```python
from build123d import *

# Parameters (mm, degrees)
SKETCH_1_R          = 12
EXTRUDE_1_DEPTH     = 19
EXTRUDE_START       = -1
SKETCH_2_R          = 2
EXTRUDE_2_DEPTH     = 1
SKETCH_3_R          = 3.5
EXTRUDE_3_DEPTH     = 1.5
SKETCH_4_R          = 2.5
EXTRUDE_4_DEPTH     = 6
CUT_EXTRUDE_START   = -5.7
CUT_EXTRUDE_1_DEPTH = 5.7
EXTRUDE_START_2     = -16.3
EXTRUDE_5_DEPTH     = 16.3
CHAMFER_1_SIZE      = 1
FILLET_1_R          = 1
CUT_EXTRUDE_2_DEPTH = 2
SKETCH_8_R          = 0.5
EXTRUDE_6_DEPTH     = 13


with BuildPart() as part:
    # Эскиз1 → Бобышка-Вытянуть1 (new body)
    with BuildSketch(Plane.XY):
        Circle(SKETCH_1_R)
    extrude(amount=EXTRUDE_1_DEPTH)

    # Эскиз2 → Бобышка-Вытянуть2 (add)
    # profile 1 of 2: a face of its own
    with BuildSketch(Plane.XY.offset(19).offset(EXTRUDE_START)):
        with BuildLine():
            Line((-15.5, 3.5), (-11.478240283, 3.5))
            ThreePointArc((-11.478240283, 3.5), (-12, 0), (-11.478240283, -3.5))
            Line((-11.478240283, -3.5), (-15.5, -3.5))
            ThreePointArc((-15.5, -3.5), (-19, 0), (-15.5, 3.5))
        make_face()
        with Locations((-15.5, 0)):
            Circle(SKETCH_2_R, mode=Mode.SUBTRACT)
    # profile 2 of 2: a face of its own
    with BuildSketch(Plane.XY.offset(19).offset(EXTRUDE_START)):
        with BuildLine():
            Line((15.5, -3.5), (11.478240283, -3.5))
            ThreePointArc((11.478240283, -3.5), (12, 0), (11.478240283, 3.5))
            Line((11.478240283, 3.5), (15.5, 3.5))
            ThreePointArc((15.5, 3.5), (19, 0), (15.5, -3.5))
        make_face()
        with Locations(Location((15.5, 0, 0), (0, 0, 180))):
            Circle(SKETCH_2_R, mode=Mode.SUBTRACT)
    extrude(amount=EXTRUDE_2_DEPTH)

    # Эскиз3 → Бобышка-Вытянуть3 (add)
    with BuildSketch(Plane.XY.offset(19)):
        with Locations((0, 6.5)):
            Circle(SKETCH_3_R)
    extrude(amount=EXTRUDE_3_DEPTH)

    # Эскиз4 → Бобышка-Вытянуть4 (add)
    with BuildSketch(Plane.XY.offset(20.5)):
        with Locations((0, 6.5)):
            Circle(SKETCH_4_R)
    extrude(amount=EXTRUDE_4_DEPTH)

    # Эскиз5 → Вырез-Вытянуть1 (cut)
    with BuildSketch(Plane.XY.offset(26.5).offset(CUT_EXTRUDE_START)):
        with BuildLine():
            Line((-1.5, 8.5), (-1.5, 4.5))
            ThreePointArc((-1.5, 4.5), (-2.5, 6.5), (-1.5, 8.5))
        make_face()
        with BuildLine():
            Line((1.5, 8.5), (1.5, 4.5))
            ThreePointArc((1.5, 4.5), (2.5, 6.5), (1.5, 8.5))
        make_face()
    extrude(amount=CUT_EXTRUDE_1_DEPTH, mode=Mode.SUBTRACT)

    # Эскиз6 → Бобышка-Вытянуть5 (add)
    with BuildSketch(Plane.XY.offset(19).offset(EXTRUDE_START_2)):
        with BuildLine():
            Line((-7.5, -16.5), (7.5, -16.5))
            Line((7.5, -16.5), (7.5, -9.367496998))
            ThreePointArc((7.5, -9.367496998), (0, -12), (-7.5, -9.367496998))
            Line((-7.5, -9.367496998), (-7.5, -16.5))
        make_face()
    extrude(amount=EXTRUDE_5_DEPTH)

    # Фаска1
    chamfer_1_edges = [part.edges().sort_by_distance(p)[0] for p in [
        (-7.5, -16.5, 10.85),
        (7.5, -16.5, 10.85),
    ]]
    chamfer(chamfer_1_edges, length=CHAMFER_1_SIZE)

    # Скругление1
    fillet_1_edges = [part.edges().sort_by_distance(p)[0] for p in [
        (-12, 0, 0),
    ]]
    fillet(fillet_1_edges, radius=FILLET_1_R)

    # Эскиз7 → Вырез-Вытянуть2 (cut)
    with BuildSketch(Plane.XZ.offset(16.5)):
        with BuildLine():
            Line((-3.5, 15.6), (3.5, 15.6))
            ThreePointArc((3.5, 15.6), (4.1, 15), (3.5, 14.4))
            Line((3.5, 14.4), (-3.5, 14.4))
            ThreePointArc((-3.5, 14.4), (-4.1, 15), (-3.5, 15.6))
        make_face()
    extrude(amount=-CUT_EXTRUDE_2_DEPTH, mode=Mode.SUBTRACT)

    # Эскиз8 → Бобышка-Вытянуть6 (add)
    with BuildSketch(Plane.XZ.offset(14.5)):
        with Locations((-2.1, 15)):
            Circle(SKETCH_8_R)
        with Locations((-1.09, 15)):
            Circle(SKETCH_8_R)
        with Locations((-0.08, 15)):
            Circle(SKETCH_8_R)
        with Locations((0.93, 15)):
            Circle(SKETCH_8_R)
        with Locations((1.94, 15)):
            Circle(SKETCH_8_R)
    extrude(amount=EXTRUDE_6_DEPTH)


solid = part.part
```
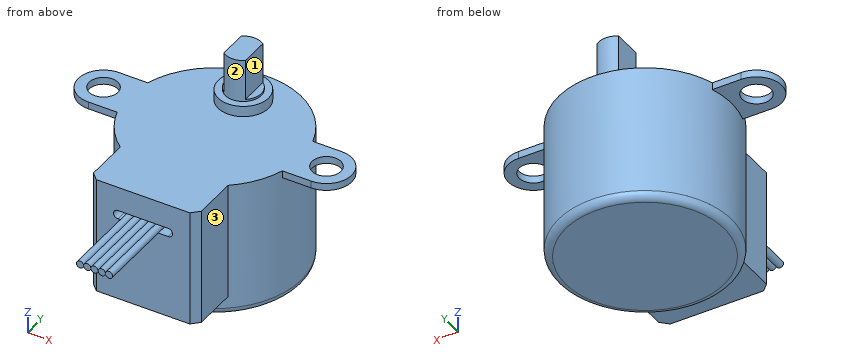
Here's how the part is built. I have some questions about the finished solid (model axes, mm). Face numbers are marked on the shaded views. A direction names the side the tool comes from. Give positions to 0.01 mm unless a question says otherwise; leave off trailing zeros. Order: outer loops, then holes, each group sorted by start corner. A loop starts at its lowest first (then second) coordinate and runs counter-clockwise, first axis right, second up. Notation, with made-up numbers: M 22,-23.75 L 65,-23.75 A5 ccw 65,-14.75 Z; hole C -12,27.25 d5. An arc over 180 degrees is marked long. Use a Markdown table: item, result. Add a question column.
1. For pin 1 Ø7.5 at (x, y) = (15, -1) entering from -Z; pin 2 Ø8 at (x, z) = (11.5, 11.5) entering from +Y; pin 3 Ø1 at (y, z) = (-8, 10.5) entering from -X; pin 4 Ø3.5 at (x, y) = (-15.5, 0) entering from +Z, each with a flat end and sliding along its axis, tell me the tip position at first contact or that it passes through.
2. I need wall thicknesses on probe 1 along Y at (x, z) = (15.5, 18.3); probe 2 along Z at (x, y) = (-2, -18); probe 3 along X at (y, z) = (4.5, 21.75). Which ranges of each line are inside material? Lowest first, please. Write a range as from..to.
3. Suppose I cut it at A-A (y = -19.5). List the corners of the cut face in (x, z) for me, and give its area (3 significant figures).
4. On a 3-axis mill with a long thin cutter (end or side, diameter ignored), from which of +Z, -Z, +X, -X, +Y, -Y can I reach the whole of each face in a straight line? I mean the marked faces 1, 2 and 3. Say none if no direction works.
5. Suppose I cut it at C-C (z = 10.25). List the corners of the cut face in (x, y) for me, and give its area (3 significant figures).
6. Suppose I cut it at D-D (y = -14). List the corners of the cut face in (x, z) for me.
Results list:
| question | item | result |
|---|---|---|
| 1 | pin 1 | stops at z = 0.04 |
| 1 | pin 2 | stops at y = 9.37 |
| 1 | pin 3 | stops at x = -9.37 |
| 1 | pin 4 | passes through |
| 2 | probe 1 | y = -3.5..-2, 2..3.5 |
| 2 | probe 2 | z = 14.51..15.49 |
| 2 | probe 3 | x = -1.5..1.5 |
| 3 | outline | C -2.1,15 d1; C -1.09,15 d1; C -0.08,15 d1; C 0.93,15 d1; C 1.94,15 d1 |
| 3 | area | 3.93 mm² |
| 4 | face 1 | +Z, +X, +Y, -Y |
| 4 | face 2 | +Z |
| 4 | face 3 | +Z, -Z, +X, -Y |
| 5 | outline | M -7.5,-15.5 L -6.5,-16.5 L 6.5,-16.5 L 7.5,-15.5 L 7.5,-9.37 A12 ccw long -7.5,-9.37 Z |
| 5 | area | 531 mm² |
| 6 | outline | M -7.5,2.7 L 7.5,2.7 L 7.5,19 L -7.5,19 Z |
